```python
from build123d import *

# Parameters (mm, degrees)
F1_DEPTH = 30
F3_DEPTH = 15
F5_DEPTH = 15
F6_W     = 5
F6_H     = 0.8216293063
F7_DEPTH = 19.0451266038


with BuildPart() as f1:
    # F0 (on Top) → F1 (new body)
    with BuildSketch(Plane.XY):
        with BuildLine():
            add(Edge.make_bspline(
                [(37.1067872729, -4.2723893299), (43.8225328786, -6.3263470576), (48.8563328981, -8.3856321871), (60, -15.0441265038)],
                knots=[0.5101508663, 0.5101508663, 0.5101508663, 0.5101508663, 1, 1, 1, 1], degree=3))
            add(Edge.make_bspline(
                [(10, 35), (12.5087825336, 25.2597781502), (9.2883909053, 8.4522198534), (30.3742546348, -1.2643312428), (37.1067872729, -4.2723893299)],
                knots=[0, 0, 0, 0, 0.494664071, 1, 1, 1, 1], degree=3))
            ThreePointArc((10, 35), (8.5355339059, 38.5355339059), (5, 40))
            Line((5, 40), (0, 40))
            Line((0, 40), (-5, 40))
            ThreePointArc((-5, 40), (-8.5355339059, 38.5355339059), (-10, 35))
            add(Edge.make_bspline(
                [(-10, 35), (-12.5087825336, 25.2597781502), (-9.2883909053, 8.4522198534), (-30.3742546348, -1.2643312428), (-37.1067872729, -4.2723893299)],
                knots=[0, 0, 0, 0, 0.494664071, 1, 1, 1, 1], degree=3))
            add(Edge.make_bspline(
                [(-37.1067872729, -4.2723893299), (-43.8225328786, -6.3263470576), (-48.8563328981, -8.3856321871), (-60, -15.0441265038)],
                knots=[0.5101508663, 0.5101508663, 0.5101508663, 0.5101508663, 1, 1, 1, 1], degree=3))
            Line((-60, -15.0441265038), (-60, -19.0441265038))
            add(Edge.make_bspline(
                [(-60, -19.0441265038), (-52.8339832092, -14.5790806997), (-35.6940193818, -5.9067861207), (-13.0268717706, -4.2301601805), (0, -4)],
                knots=[0, 0, 0, 0, 0.4618585351, 1, 1, 1, 1], degree=3))
            add(Edge.make_bspline(
                [(60, -19.0441265038), (52.8339832092, -14.5790806997), (35.6940193818, -5.9067861207), (13.0268717706, -4.2301601805), (0, -4)],
                knots=[0, 0, 0, 0, 0.4618585351, 1, 1, 1, 1], degree=3))
            Line((60, -19.0441265038), (60, -15.0441265038))
        make_face()
    extrude(amount=F1_DEPTH)

    # F2 (on face) → F3 (cut)
    with BuildSketch(Plane.XY.offset(30)):
        Polygon((15, 40), (-15, 40), (-15, 13.6816753075), (-6.9741668392, -8.3691200741), (7.0873022438, -8.3691200741), (15, 13.3708383381), align=None)
    extrude(amount=-F3_DEPTH, mode=Mode.SUBTRACT)

    # F4 (on face) → F5 (cut, through all)
    with BuildSketch(Plane.XY.offset(15)):
        with BuildLine():
            Line((0.5, 33.355844829), (-0.5, 33.355844829))
            ThreePointArc((-0.5, 33.355844829), (-1.9142135624, 32.7700583913), (-2.5, 31.355844829))
            Line((-2.5, 31.355844829), (-2.5, 11.5851387382))
            Line((-2.5, 11.5851387382), (2.5, 11.5851387382))
            Line((2.5, 11.5851387382), (2.5, 31.355844829))
            ThreePointArc((2.5, 31.355844829), (1.9142135624, 32.7700583913), (0.5, 33.355844829))
        make_face()
    extrude(amount=-F5_DEPTH, mode=Mode.SUBTRACT)

    # F6 (on Front) → F7 (cut, through all)
    with BuildSketch(Plane.XZ):
        with Locations((57.5, 0.4108146532)):
            Rectangle(F6_W, F6_H)
    extrude(amount=F7_DEPTH, mode=Mode.SUBTRACT)


solid = f1.part
```
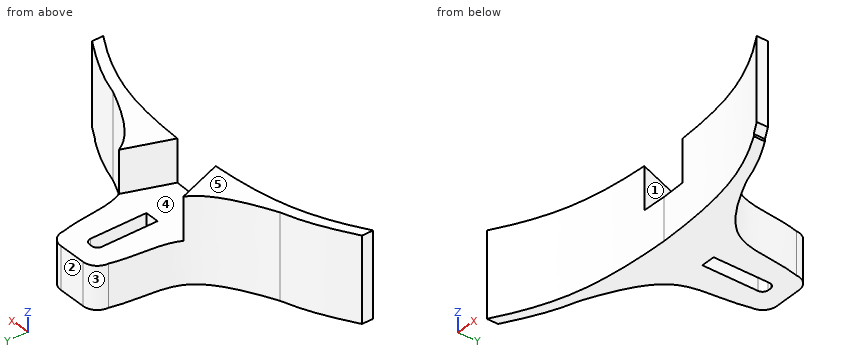
Source: CAD feature listing. Evaluate the final solid. Frame: model axes, mm. Face numbers are marked on the shaded views. A direction names the side the tool comes from. Give positions to 0.01 mm unless a question says otherwise; leave off trailing zeros. Use a Markdown table: item, result. Add a question column.
(1) Ray query, line 1 (X direction, y = -12, z = 8.5); line 2 (X direction, y = 33, z = 10.5); line 3 (Y direction, x = 55, z = 20). Return the intervals inside material, ascending.
(2) First-contact query: pin 1 Ø2 at (y, z) = (-0.5, 8) entering from +X; pin 2 Ø1 at (y, z) = (-12.5, 26.5) entering from +X; pin 3 Ø7.5 at (y, z) = (20, 4.5) entering from -X. Flat tips, straight axial feed; report the tip coordinate or a pass-through.
(3) Access query for the marked faces 4 and 5. Directions: +Z, -Z, +X, -X, +Y, -Y. A direction counts if a zero-diameter tool reaches every point of the face in a straight line with its end or side. Return the directions, or none.
(4) Pull-direction query (X, two-part tool) for the marked faces 1, 2 and 3; classes: +X half, -X half, draft (parallel to the pull), parting line (faces both ways), or undercut.
Checked values:
| question | item | result |
|---|---|---|
| 1 | line 1 | -54.76 to -46.83, 46.83 to 54.76 |
| 1 | line 2 | -10.46 to -1.64, 1.64 to 10.46 |
| 1 | line 3 | -16.09 to -12.13 |
| 2 | pin 1 | x = 31.15 |
| 2 | pin 2 | x = 56.52 |
| 2 | pin 3 | x = -12.8 |
| 3 | face 4 | +Z, +Y |
| 3 | face 5 | +Z, +X, -X, +Y, -Y |
| 4 | face 1 | undercut |
| 4 | face 2 | draft |
| 4 | face 3 | -X half |
